from build123d import *

# Parameters (mm, degrees)
BOSS_EXTRUDE1_DEPTH = 1.6
SKETCH2_R           = 0.5
CUT_EXTRUDE1_DEPTH  = 16.734039532


with BuildPart() as part:
    # Sketch1 → Boss-Extrude1 (new body)
    with BuildSketch(Plane.XY):
        Polygon((7, 11.46), (5.6, 11.46), (5.6, 4.66), (7, 4.66), (7, -0.732), (5.6, -0.732), (5.6, -7.532), (7, -7.532), (7, -14), (-7, -14), (-7, 14), (7, 14), align=None)
    extrude(amount=BOSS_EXTRUDE1_DEPTH)

    # Sketch2 → Cut-Extrude1 (cut, through all)
    with BuildSketch(Plane.XY.offset(1.6)):
        with Locations((-2.486935959, 13.013337482)):
            Circle(SKETCH2_R)
        with Locations((-2.486935959, 10.558296047)):
            Circle(SKETCH2_R)
        with Locations((-2.486935959, 8.103254612)):
            Circle(SKETCH2_R)
        with Locations((-2.486935959, 5.648213177)):
            Circle(SKETCH2_R)
        with Locations((-2.486935959, 3.193171742)):
            Circle(SKETCH2_R)
        with Locations((-2.486935959, 0.738130307)):
            Circle(SKETCH2_R)
        with Locations((-2.486935959, -1.716911128)):
            Circle(SKETCH2_R)
        with Locations((-2.486935959, -6.626993998)):
            Circle(SKETCH2_R)
        with Locations((-2.486935959, -9.082035433)):
            Circle(SKETCH2_R)
        with Locations((2.527644678, -4.171952563)):
            Circle(SKETCH2_R)
        with Locations((2.527644678, 8.103254612)):
            Circle(SKETCH2_R)
        with Locations((-2.486935959, -4.171952563)):
            Circle(SKETCH2_R)
        with Locations((2.527644678, 0.738130307)):
            Circle(SKETCH2_R)
        with Locations((2.527644678, 3.193171742)):
            Circle(SKETCH2_R)
        with Locations((5.034934997, 3.193171742)):
            Circle(SKETCH2_R)
        with Locations((5.034934997, 0.738130307)):
            Circle(SKETCH2_R)
        with Locations((2.527644678, 13.013337482)):
            Circle(SKETCH2_R)
        with Locations((5.034934997, 13.013337482)):
            Circle(SKETCH2_R)
        with Locations((5.034934997, -9.082035433)):
            Circle(SKETCH2_R)
        with Locations((2.527644678, -9.082035433)):
            Circle(SKETCH2_R)
    extrude(amount=-CUT_EXTRUDE1_DEPTH, mode=Mode.SUBTRACT)


solid = part.part
Input: part model. Units: mm. Frame: model coordinates. A direction names the side the tool comes from. Round coordinates to 2 decimals unless told otherwise and drop trailing zeros.
1) Contact query for a flat-ended pin moving along its axis: P1, Ø0.5, axis at y = 7, z = 0.5, coming from the +X side. Output: stop coordinate, or through.
2) Reachability of faces 4 (the flat face through (6, 4.66, 1)), 5 (the cylindrical face through (-2.55, 3.69, 0.81)) from +Z, -Z, +X, -X, +Y, -Y: full face, straight path, thin tool, end or side. Return the list, or none.
3) Ray query, L1, parallel to Y at x = 6.5, z = 1.05; L2, parallel to X at y = 3.5, z = 0.4; L3, parallel to Y at x = 4.75, z = 0.5. Return the intervals inside material, ascending.
4) Draft query along Y for faces 1 (the flat face through (0, 14, 1)), 2 (the cylindrical face through (2.16, 13.35, 0.81)), 3 (the flat face through (7, 13, 1)). Return one class per face: pulls with the +Y half, pulls with the -Y half, needs draft (parallel to the pull), parting line crosses it, or undercut.
5) Cut plane A-A (z = 1.15). Count the separate pieces of the cut face and the enclosed holes in it, then the cut area to 3 significant figures.
Geometry says:
1. P1: stops at x = 5.6
2. face 4: +Z, -Z, +X
2. face 5: +Z, -Z
3. L1: y = -14 to -7.53, -0.73 to 4.66, 11.46 to 14
3. L2: x = -7 to -2.88, -2.09 to 2.13, 2.92 to 4.64, 5.43 to 7
3. L3: y = -14 to -9.49, -8.67 to 0.33, 1.15 to 2.78, 3.6 to 12.6, 13.42 to 14
4. face 1: pulls with the +Y half
4. face 2: undercut
4. face 3: needs draft
5. separate pieces: 1
5. enclosed holes: 20
5. area: 357 mm2
